The model under review builds one solid part; all positions refer to its coordinate system, in mm. Face numbers are marked on the shaded views. A direction names the side the tool comes from. Coordinates: 2 decimals unless noted, no trailing zeros. Write each loop counter-clockwise with the first axis right and the second up, starting at its lowest first coordinate (ties: lowest second). Pieces come first, ordered by that corner, then holes. Notation, with made-up numbers: (-33, 0.25) - (20, 0.25) arc R27 cw to (20, 25.25) - close; hole circle Ø9 at (46.5, 32). An arc over 180 degrees is marked (long way). Put each result on its own line as item: value.
from build123d import *

# Parameters (mm, degrees)
SKETCH2_W               = 31.75
SKETCH2_H               = 31.75
BOSS_EXTRUDE2_DEPTH     = 19.05
CUT_EXTRUDE1_DEPTH      = 30.443738723
CUT_EXTRUDE1_DEPTH_BACK = 30.443738723
SKETCH4_W               = 19.05
SKETCH4_H               = 19.05
CUT_EXTRUDE2_DEPTH      = 30.443738723
CUT_EXTRUDE2_DEPTH_BACK = 30.443738723
SKETCH5_W               = 19.05
SKETCH5_H               = 6.35
CUT_EXTRUDE3_DEPTH      = 30.443738723
CUT_EXTRUDE3_DEPTH_BACK = 30.443738723


with BuildPart() as part:
    # Sketch2 → Boss-Extrude2 (new, symmetric)
    with BuildSketch(Plane(origin=(0, 0, 0), x_dir=(0, 0, -1), z_dir=(1, 0, 0))):
        Rectangle(SKETCH2_W, SKETCH2_H)
    extrude(amount=BOSS_EXTRUDE2_DEPTH, both=True)

    # Sketch4 → Cut-Extrude1 (cut, two sides: drawn at the far end of the back side and taken through both)
    with BuildSketch(Plane(origin=(0, 0, 0), x_dir=(0, 0, -1), z_dir=(1, 0, 0)).offset(-CUT_EXTRUDE1_DEPTH_BACK)):
        with Locations((0, 6.35)):
            Rectangle(SKETCH4_W, SKETCH4_H)
    extrude(amount=CUT_EXTRUDE1_DEPTH + CUT_EXTRUDE1_DEPTH_BACK, mode=Mode.SUBTRACT)

    # Sketch5 → Cut-Extrude2 (cut, two sides: drawn at the far end of the back side and taken through both)
    with BuildSketch(Plane(origin=(0, 0, 0), x_dir=(0, 0, -1), z_dir=(1, 0, 0)).offset(-CUT_EXTRUDE2_DEPTH_BACK)):
        with Locations((0, -12.7)):
            Rectangle(SKETCH5_W, SKETCH5_H)
    extrude(amount=CUT_EXTRUDE2_DEPTH + CUT_EXTRUDE2_DEPTH_BACK, mode=Mode.SUBTRACT)

    # Sketch6 → Cut-Extrude3 (cut, two sides: drawn at the far end of the back side and taken through both)
    with BuildSketch(Plane.XY.offset(-CUT_EXTRUDE3_DEPTH_BACK)):
        Polygon((19.05, 15.875), (19.05, 3.175), (-6.35, 15.875), align=None)
    extrude(amount=CUT_EXTRUDE3_DEPTH + CUT_EXTRUDE3_DEPTH_BACK, mode=Mode.SUBTRACT)


solid = part.part
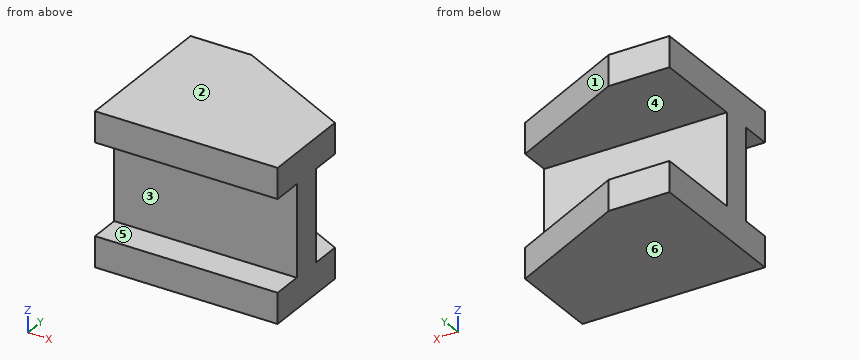
1. For pin 1 Ø1 at (x, z) = (14.5, 6) entering from +Y (3 decimals); pin 2 Ø8 at (x, z) = (-9, -9) entering from -Y (3 decimals), all flat-tipped, find the tip position at first contact; note any pin that passes through.
Determined:
pin 1: stops at y = -3.175
pin 2: stops at y = -15.875
2. Consider section C-C on z = -14. State the section outline as (x, y) points (3 decimals).
Determined:
outline: (-19.05, -15.875) - (19.05, -15.875) - (19.05, 3.175) - (-6.35, 15.875) - (-19.05, 15.875) - close
3. Consider section D-D on y = -11. State the section outline as (x, z) points (3 decimals), plus the area to 3 significant figures.
Determined:
outline: (-19.05, -15.875) - (19.05, -15.875) - (19.05, -9.525) - (-19.05, -9.525) - close; (-19.05, 9.525) - (19.05, 9.525) - (19.05, 15.875) - (-19.05, 15.875) - close
area: 484 mm^2
4. The part is to be moulded in two halves that separate along Z. For the marked faces 1, 2 and 3, say which applies: +Z half, -Z half, draft (parallel to the pull), parting line (faces both ways), or undercut.
Determined:
face 1: draft
face 2: +Z half
face 3: undercut
5. To check wall thickness, follow probe 1 along Z at (x, y) = (1, -10) (3 decimals); probe 2 along Y at (x, z) = (8, 2.5) (3 decimals); probe 3 along X at (y, z) = (13, 12). State the ranges of each line that lie inside material, in increasing order.
Determined:
probe 1: z = -15.875 to -9.525, 9.525 to 15.875
probe 2: y = -9.525 to -3.175
probe 3: x = -19.05 to -0.6
6. Consider section A-A on y = 9.5. State the section outline as (x, z) points (3 decimals), plus the area to 3 significant figures.
Determined:
outline: (-19.05, -15.875) - (6.4, -15.875) - (6.4, -9.525) - (-19.05, -9.525) - close; (-19.05, 9.525) - (6.4, 9.525) - (6.4, 15.875) - (-19.05, 15.875) - close
area: 323 mm^2
7. Machinability: for the marked faces 4, 5 and 6, which of the approach directions +Z, -Z, +X, -X, +Y, -Y give a long, thin tool a straight path to every point of the face, cutting with its end or side? Answer none if there is none.
Determined:
face 4: +X, -X, +Y
face 5: +X, -X, -Y
face 6: -Z, +X, -X, +Y, -Y
8. Consider section B-B on x = -3. State the section outline as (y, z) points (3 decimals).
Determined:
outline: (-15.875, -15.875) - (14.2, -15.875) - (14.2, -9.525) - (-3.175, -9.525) - (-3.175, 9.525) - (14.2, 9.525) - (14.2, 15.875) - (-15.875, 15.875) - (-15.875, 9.525) - (-9.525, 9.525) - (-9.525, -9.525) - (-15.875, -9.525) - close
